Input: part model. Units: mm. Frame: model coordinates. A direction names the side the tool comes from. Round coordinates to 2 decimals unless told otherwise and drop trailing zeros. Loops run counter-clockwise (first coordinate to the right, second up) from the corner with the lowest first, then second, coordinate; pieces in that order, holes last. Notation, with made-up numbers: M -22,-36.75 L 16,-36.75 A15 ccw 16,-24.75 Z; hole C -5,-10 d8. An arc over 180 degrees is marked long. Put each result on its own line as item: value. Start each with the question number.
1) Section A-A on z = 0. Output: boundary loops of the cut face in (x, y) (3 decimals), plus the area to 3 significant figures.
2) Reachability of faces 4 (the face through (17, -2.54, -17)), 5 (the face through (17, 0, -17)), 6 (the face through (-14.351, -1, 0)) from +Z, -Z, +X, -X, +Y, -Y: full face, straight path, thin tool, end or side. Return the list, or none.
3) Pin query (flat end, axial travel): pin 1 (4 mm diameter, centred on y = -26, z = 6, fed in from -X); pin 2 (10 mm diameter, centred on y = -39.5, z = 32, fed in from -X); pin 3 (8 mm diameter, centred on y = -40, z = 12, fed in from +X); pin 4 (2.5 mm diameter, centred on x = -17.73, z = 0, fed in from -Y). Return the tip coordinate at first contact, or that it passes through.
4) Section C-C on y = -20.5. Output: boundary loops of the cut face in (x, z) (3 decimals).
5) Section B-B on x = 0. Output: boundary loops of the cut face in (y, z) (3 decimals), plus the area to 3 significant figures.
6) Line query: probe 1 along Z at (x, y) = (0, -39.5) (3 decimals); probe 2 along X at (y, z) = (-31.5, 7); probe 3 along X at (y, z) = (-48, 10). Output: solid intervals per line, ascending.
7) Draft query along Z for faces 1 (the face through (36.5, -51.435, -15.1)), 2 (the face through (-5.11, -26.65, 38.91)), 3 (the face through (-8.948, -26.645, -40.293)). Return one class per face: +Z half, -Z half, draft (parallel to the pull), parting line (faces both ways), or undercut.
from build123d import *

# Parameters (mm, degrees)
F0_R          = 41.275
F1_DEPTH      = 2.54
F3_R          = 41.275
F3_R_2        = 39.243
F4_DEPTH      = 48.895
F5_R          = 2.54
F2_R          = 1.905
F6_DEPTH      = 25.4
F6_DEPTH_BACK = 25.4
F7_R          = 2.54


with BuildPart() as f1:
    # F0 (on Front) → F1 (new body)
    with BuildSketch(Plane.XZ):
        Circle(F0_R)
    extrude(amount=F1_DEPTH)

    # F3 (on face) → F4 (join)
    with BuildSketch(Plane.XZ.offset(2.54)):
        Circle(F3_R)
        Circle(F3_R_2, mode=Mode.SUBTRACT)
    extrude(amount=F4_DEPTH)

    # F5
    f5_edges = [f1.edges().sort_by_distance(p)[0] for p in [
        (-41.275, 0, 0),
    ]]
    fillet(f5_edges, radius=F5_R)

    # F2 (on face) → F6 (cut, two sides)
    with BuildSketch(Plane.XZ.offset(2.54)) as f6_sk:
        with Locations((17.5006, 0)):
            Circle(F2_R)
        with Locations((-17.7292, 0)):
            Circle(F2_R)
        with BuildLine():
            Line((14.351, 3.81), (20.3473659475, 3.81))
            ThreePointArc((20.3473659475, 3.81), (0, 20.701), (-20.3473659475, 3.81))
            Line((-20.3473659475, 3.81), (-14.351, 3.81))
            Line((-14.351, 3.81), (-14.351, -3.81))
            Line((-14.351, -3.81), (-20.3473659475, -3.81))
            ThreePointArc((-20.3473659475, -3.81), (0, -20.701), (20.3473659475, -3.81))
            Line((20.3473659475, -3.81), (14.351, -3.81))
            Line((14.351, -3.81), (14.351, 3.81))
        make_face()
    extrude(amount=-F6_DEPTH, mode=Mode.SUBTRACT)
    extrude(f6_sk.sketch, amount=F6_DEPTH_BACK, mode=Mode.SUBTRACT)

    # F7
    f7_edges = [f1.edges().sort_by_distance(p)[0] for p in [
        (-20.347366, -1.27, 3.81),
        (-14.351, -1.27, 3.81),
        (-14.351, -1.27, -3.81),
        (-20.347366, -1.27, -3.81),
        (14.351, -1.27, 3.81),
        (14.351, -1.27, -3.81),
        (20.347366, -1.27, -3.81),
        (20.347366, -1.27, 3.81),
    ]]
    fillet(f7_edges, radius=F7_R)


solid = f1.part
Geometry results:
1. outline: M -41.275,-51.435 L -39.243,-51.435 L -39.243,-2.54 L -19.634,-2.54 L -19.634,0 L -38.735,0 A2.54 ccw -41.275,-2.54 Z; M -15.824,-2.54 L -14.351,-2.54 L -14.351,0 L -15.824,0 Z; M 14.351,-2.54 L 15.596,-2.54 L 15.596,0 L 14.351,0 Z; M 19.406,-2.54 L 39.243,-2.54 L 39.243,-51.435 L 41.275,-51.435 L 41.275,-2.54 A2.54 ccw 38.735,0 L 19.406,0 Z
1. area: 313 mm²
2. face 4: -Y
2. face 5: +Z, -Z, +X, -X, +Y
2. face 6: +Y, -Y
3. pin 1: stops at x = -41.08
3. pin 2: stops at x = -31.22
3. pin 3: stops at x = 40.49
3. pin 4: passes through
4. outline: C 0,0 d82.55; hole C 0,0 d78.486
5. outline: M -51.435,-41.275 L -2.54,-41.275 A2.54 ccw 0,-38.735 L 0,-20.701 L -2.54,-20.701 L -2.54,-39.243 L -51.435,-39.243 Z; M -51.435,39.243 L -2.54,39.243 L -2.54,20.701 L 0,20.701 L 0,38.735 A2.54 ccw -2.54,41.275 L -51.435,41.275 Z
5. area: 300 mm²
6. probe 1: z = -41.275 to -39.243, 39.243 to 41.275
6. probe 2: x = -40.68 to -38.61, 38.61 to 40.68
6. probe 3: x = -40.05 to -37.95, 37.95 to 40.05
7. face 1: draft
7. face 2: undercut
7. face 3: parting line
